```python
from build123d import *

# Parameters (mm, degrees)
SKETCH1_R            = 25
BOSS_EXTRUDE2_DEPTH  = 3
SKETCH3_R            = 38
BOSS_EXTRUDE4_DEPTH  = 2
SKETCH5_R            = 32
SKETCH5_R_2          = 27
BOSS_EXTRUDE5_DEPTH  = 6
SKETCH6_R            = 5
BOSS_EXTRUDE7_DEPTH  = 6
SKETCH7_R            = 38
BOSS_EXTRUDE9_DEPTH  = 2
FILLET2_R            = 2
FILLET3_R            = 2
FILLET5_R            = 2
SKETCH8_R            = 30
BOSS_EXTRUDE10_DEPTH = 9
CUT_EXTRUDE1_DEPTH   = 10
CUT_EXTRUDE3_DEPTH   = 10


with BuildPart() as part:
    # Sketch1 → Boss-Extrude2 (new body)
    with BuildSketch(Plane(origin=(0, 0, 0), x_dir=(1, 0, 0), z_dir=(0, 1, 0))):
        Circle(SKETCH1_R)
        with BuildLine():
            Line((20, -3.5), (7.537849637, -5))
            ThreePointArc((7.537849637, -5), (6.396060395, -6.396060395), (5, -7.537849637))
            Line((5, -7.537849637), (3.5, -20))
            Line((3.5, -20), (-3.5, -20))
            Line((-3.5, -20), (-5, -7.537849637))
            ThreePointArc((-5, -7.537849637), (-6.396060395, -6.396060395), (-7.537849637, -5))
            Line((-7.537849637, -5), (-20, -3.5))
            Line((-20, -3.5), (-20, 3.5))
            Line((-20, 3.5), (-7.537849637, 5))
            ThreePointArc((-7.537849637, 5), (-6.396060395, 6.396060395), (-5, 7.537849637))
            Line((-5, 7.537849637), (-3.5, 20))
            Line((-3.5, 20), (3.5, 20))
            Line((3.5, 20), (5, 7.537849637))
            ThreePointArc((5, 7.537849637), (6.396060395, 6.396060395), (7.537849637, 5))
            Line((7.537849637, 5), (20, 3.5))
            Line((20, 3.5), (20, -3.5))
        make_face(mode=Mode.SUBTRACT)
    extrude(amount=BOSS_EXTRUDE2_DEPTH)

    # Sketch3 → Boss-Extrude4 (add)
    with BuildSketch(Plane(origin=(0, 3, 0), x_dir=(1, 0, 0), z_dir=(0, 1, 0))):
        Circle(SKETCH3_R)
    extrude(amount=BOSS_EXTRUDE4_DEPTH)

    # Sketch5 → Boss-Extrude5 (add)
    with BuildSketch(Plane(origin=(0, 5, 0), x_dir=(1, 0, 0), z_dir=(0, 1, 0))):
        Circle(SKETCH5_R)
        Circle(SKETCH5_R_2, mode=Mode.SUBTRACT)
    extrude(amount=BOSS_EXTRUDE5_DEPTH)

    # Sketch6 → Boss-Extrude7 (add)
    with BuildSketch(Plane(origin=(0, 5, 0), x_dir=(1, 0, 0), z_dir=(0, 1, 0))):
        Circle(SKETCH6_R)
    extrude(amount=BOSS_EXTRUDE7_DEPTH)

    # Sketch7 → Boss-Extrude9 (add)
    with BuildSketch(Plane(origin=(0, 11, 0), x_dir=(1, 0, 0), z_dir=(0, 1, 0))):
        Circle(SKETCH7_R)
    extrude(amount=BOSS_EXTRUDE9_DEPTH)

    # Fillet2
    fillet2_edges = [part.edges().sort_by_distance(p)[0] for p in [
        (-32, 11, 0),
    ]]
    fillet(fillet2_edges, radius=FILLET2_R)

    # Fillet3
    fillet3_edges = [part.edges().sort_by_distance(p)[0] for p in [
        (-32, 5, 0),
    ]]
    fillet(fillet3_edges, radius=FILLET3_R)

    # Fillet5
    fillet5_edges = [part.edges().sort_by_distance(p)[0] for p in [
        (-25, 3, 0),
    ]]
    fillet(fillet5_edges, radius=FILLET5_R)

    # Sketch8 → Boss-Extrude10 (add)
    with BuildSketch(Plane(origin=(0, 13, 0), x_dir=(1, 0, 0), z_dir=(0, 1, 0))):
        Circle(SKETCH8_R)
    extrude(amount=-BOSS_EXTRUDE10_DEPTH)

    # Sketch9 → Cut-Extrude1 (cut)
    with BuildSketch(Plane(origin=(0, 13, 0), x_dir=(1, 0, 0), z_dir=(0, 1, 0))):
        with BuildLine():
            Line((5, -5), (5, -29.580398915))
            ThreePointArc((5, -29.580398915), (21.213203436, -21.213203436), (29.580398915, -5))
            Line((29.580398915, -5), (5, -5))
        make_face()
        with BuildLine():
            Line((-5, -29.580398915), (-5, -5))
            Line((-5, -5), (-29.580398915, -5))
            ThreePointArc((-29.580398915, -5), (-21.213203436, -21.213203436), (-5, -29.580398915))
        make_face()
        with BuildLine():
            Line((-29.580398915, 5), (-5, 5))
            Line((-5, 5), (-5, 29.580398915))
            ThreePointArc((-5, 29.580398915), (-21.213203436, 21.213203436), (-29.580398915, 5))
        make_face()
        with BuildLine():
            ThreePointArc((29.580398915, 5), (21.213203436, 21.213203436), (5, 29.580398915))
            Line((5, 29.580398915), (5, 5))
            Line((5, 5), (29.580398915, 5))
        make_face()
    extrude(amount=-CUT_EXTRUDE1_DEPTH, mode=Mode.SUBTRACT)

    # Sketch10 → Cut-Extrude3 (cut)
    with BuildSketch(Plane(origin=(0, 3, 0), x_dir=(-1, 0, 0), z_dir=(0, -1, 0))):
        with BuildLine():
            ThreePointArc((-9.154882095, 6.256063873), (-7.840900748, 7.840311015), (-6.256752441, 9.154411518))
            Line((-6.256752441, 9.154411518), (-5.984311052, 20.129282681))
            ThreePointArc((-5.984311052, 20.129282681), (-14.874716269, 14.823724765), (-20.149713772, 5.915152991))
            Line((-20.149713772, 5.915152991), (-9.154882095, 6.256063873))
        make_face()
        with BuildLine():
            Line((5.984311052, 20.129282681), (6.256752441, 9.154411518))
            ThreePointArc((6.256752441, 9.154411518), (7.840900748, 7.840311015), (9.154882095, 6.256063873))
            Line((9.154882095, 6.256063873), (20.149713772, 5.915152991))
            ThreePointArc((20.149713772, 5.915152991), (14.874716269, 14.823724765), (5.984311052, 20.129282681))
        make_face()
        with BuildLine():
            Line((20.149713772, -5.915152991), (9.154882095, -6.256063873))
            ThreePointArc((9.154882095, -6.256063873), (7.840900748, -7.840311015), (6.256752441, -9.154411518))
            Line((6.256752441, -9.154411518), (5.984311052, -20.129282681))
            ThreePointArc((5.984311052, -20.129282681), (14.874716269, -14.823724765), (20.149713772, -5.915152991))
        make_face()
        with BuildLine():
            ThreePointArc((-6.256752441, -9.154411518), (-7.840900748, -7.840311015), (-9.154882095, -6.256063873))
            Line((-9.154882095, -6.256063873), (-20.149713772, -5.915152991))
            ThreePointArc((-20.149713772, -5.915152991), (-14.874716269, -14.823724765), (-5.984311052, -20.129282681))
            Line((-5.984311052, -20.129282681), (-6.256752441, -9.154411518))
        make_face()
    extrude(amount=CUT_EXTRUDE3_DEPTH, mode=Mode.SUBTRACT)


solid = part.part
```
The listing builds one solid part. Answer for the finished solid, in the listing's coordinates (mm). A direction names the side the tool comes from. Round coordinates to 2 decimals unless told otherwise and drop trailing zeros. Loops run counter-clockwise (first coordinate to the right, second up) from the corner with the lowest first, then second, coordinate; pieces in that order, holes last.
Q1. Which of the six approach directions +Z, -Z, +X, -X, +Y, -Y give full straight-line access (tool end or side, diameter ignored) to faces 1 (the face through (-1, 13, -1)), 2 (the face through (16, 3, 16)), 3 (the face through (-28, 11, 20)), 4 (the face through (0, 1, 20)), 5 (the face through (-7.82, 1.52, -7.86))?
Q2. For a pull along X with two mould halves and no side action, classify faces 6 (the face through (4.26, 1.48, 13.68)), 7 (the face through (5, 0, 11)) as released by +X, released by -X, zero draft, split by the parting line, or undercut.
Q3. Given pin 1 Ø3 at (y, z) = (7, 15) entering from +X; pin 2 Ø1.5 at (y, z) = (3.5, 16.5) entering from -X; pin 3 Ø3 at (x, z) = (-1, 28.5) entering from -Y, each flat-ended and moving along its own axis, determine where each tip first touches the part or whether it passes through.
Q4. Section D-D, the plane z = -14.5 is taken. Count the separate pieces of the cut face and the enclosed holes in it, then the cut area to 3 significant figures.
Q5. Section B-B, the plane z = 0 is taken. Determine the outline of the cut face in (x, y), then the cut area to 3 significant figures.
Q6. Find the intervals of material crossed by line 1 (Z direction, x = 7, y = 10.5); line 2 (X direction, y = 5.75, z = -6.5); line 3 (X direction, y = 7.5, z = 18.5), in increasing order.
Q7. Section C-C, the plane x = 0 is taken. Determine the outline of the cut face in (y, z), then the cut area to 3 significant figures.
Q8. Section A-A, the plane y = 6 is taken. Determine the outline of the cut face in (x, z).
Completed:
1. face 1: +Z, -Z, +X, -X, +Y
1. face 2: +Y
1. face 3: none
1. face 4: -Y
1. face 5: +Y, -Y
2. face 6: undercut
2. face 7: zero draft
3. pin 1: stops at x = 29.19
3. pin 2: stops at x = -34.58
3. pin 3: stops at y = 3
4. separate pieces: 5
4. enclosed holes: 0
4. area: 247 mm2
5. outline: (-38, 3) - (-27, 3) arc R2 cw to (-25, 1) - (-25, 0) - (-20, 0) - (-20, 3) - (20, 3) - (20, 0) - (25, 0) - (25, 1) arc R2 cw to (27, 3) - (38, 3) - (38, 5) - (34, 5) arc R2 cw to (32, 7) - (32, 9) arc R2 cw to (34, 11) - (38, 11) - (38, 13) - (-38, 13) - (-38, 11) - (-34, 11) arc R2 cw to (-32, 9) - (-32, 7) arc R2 cw to (-34, 5) - (-38, 5) - close
5. area: 723 mm2
6. line 1: z = -31.92 to -29.17, -5 to 5, 29.17 to 31.92
6. line 2: x = -31.78 to -29.29, -5 to 5, 29.29 to 31.78
6. line 3: x = -26.11 to -23.62, -5 to 5, 23.62 to 26.11
7. outline: (0, -25) - (1, -25) arc R2 cw to (3, -27) - (3, -38) - (5, -38) - (5, -34) arc R2 cw to (7, -32) - (9, -32) arc R2 cw to (11, -34) - (11, -38) - (13, -38) - (13, 38) - (11, 38) - (11, 34) arc R2 cw to (9, 32) - (7, 32) arc R2 cw to (5, 34) - (5, 38) - (3, 38) - (3, 27) arc R2 cw to (1, 25) - (0, 25) - (0, 20) - (3, 20) - (3, -20) - (0, -20) - close
7. area: 723 mm2
8. outline: circle Ø64.54 at (0, 0); hole (-29.58, -5) arc R30 ccw to (-5, -29.58) - (-5, -5) - close; hole (-29.58, 5) - (-5, 5) - (-5, 29.58) arc R30 ccw to start; hole (5, -29.58) arc R30 ccw to (29.58, -5) - (5, -5) - close; hole (5, 5) - (29.58, 5) arc R30 ccw to (5, 29.58) - close
